from build123d import *

# Parameters (mm, degrees)
F0_W     = 19.05
F0_H     = 254
F1_DEPTH = 19.05
F0_W_2   = 241.3
F2_DEPTH = 12.7


with BuildPart() as f1:
    # F0 (on Front) → F1 (new body)
    with BuildSketch(Plane.XZ):
        with Locations((-269.875, 0)):
            Rectangle(F0_W, F0_H)
    extrude(amount=F1_DEPTH)



with BuildPart() as f1b:
    # F0 (on Front) → F1, piece 2 (new body)
    with BuildSketch(Plane.XZ):
        with Locations((-120.65, 0)):
            Rectangle(F0_W_2, F0_H)
        with Locations((120.65, 0)):
            Rectangle(F0_W_2, F0_H)
    extrude(amount=F1_DEPTH)


with BuildPart() as f1c:
    # F0 (on Front) → F1, piece 3 (new body)
    with BuildSketch(Plane.XZ):
        with Locations((269.875, 0)):
            Rectangle(F0_W, F0_H)
    extrude(amount=F1_DEPTH)


with BuildPart() as f1_1:
    add(f1.part)

    add(f1b.part)  # F2 merges F1b

    add(f1c.part)  # F2 merges F1c
    # F0 (on Front) → F2 (join)
    with BuildSketch(Plane.XZ):
        with Locations((-250.825, 0)):
            Rectangle(F0_W, F0_H)
        with Locations((250.825, 0)):
            Rectangle(F0_W, F0_H)
    extrude(amount=F2_DEPTH)


solid = f1_1.part
Verification items for the finished model (mm, model axes). A direction names the side the tool comes from. Coordinates: 2 decimals unless noted, no trailing zeros. Write each loop counter-clockwise with the first axis right and the second up, starting at its lowest first coordinate (ties: lowest second). Pieces come first, ordered by that corner, then holes. Notation, with made-up numbers: M -10,-31 L 39,-31 A21 ccw 39,-18 Z; hole C -33,-17 d10. An arc over 180 degrees is marked long. Use a Markdown table: item, result.
Q1. Thickness scan on line 1 (X direction, y = -14.25, z = 79); line 2 (Y direction, x = 243.5, z = -34.5). Record the ranges inside material, lowest first.
Reply:
| item | result |
|---|---|
| line 1 | x = -279.4 to -260.35, -241.3 to 241.3, 260.35 to 279.4 |
| line 2 | y = -12.7 to 0 |
Q2. Draft check along X on faces 3 (the face through (-279.4, -9, -2)), 4 (the face through (-251, -12.7, 2)), 5 (the face through (-3, -19.05, 2)). Enter one of: +X half, -X half, draft (parallel to the pull), parting line (faces both ways), or undercut.
Reply:
| item | result |
|---|---|
| face 3 | -X half |
| face 4 | undercut |
| face 5 | draft |
Q3. Sectioned sample at A-A, the plane y = -16. Record the boundary of the cut face in (x, z).
Reply:
| item | result |
|---|---|
| outline | M -279.4,-127 L -260.35,-127 L -260.35,127 L -279.4,127 Z; M -241.3,-127 L 241.3,-127 L 241.3,127 L -241.3,127 Z; M 260.35,-127 L 279.4,-127 L 279.4,127 L 260.35,127 Z |
Q4. Set-up check for faces 1 (the face through (251, -12.7, 2)), 2 (the face through (-4, -9, 127)): record each of +Z, -Z, +X, -X, +Y, -Y from which the full face is reachable in a straight line by a thin tool's end or side.
Reply:
| item | result |
|---|---|
| face 1 | +Z, -Z, -Y |
| face 2 | +Z, +X, -X, +Y, -Y |
Q5. Sectioned sample at B-B, the plane z = 66.5. Record the boundary of the cut face in (x, y).
Reply:
| item | result |
|---|---|
| outline | M -279.4,-19.05 L -260.35,-19.05 L -260.35,-12.7 L -241.3,-12.7 L -241.3,-19.05 L 241.3,-19.05 L 241.3,-12.7 L 260.35,-12.7 L 260.35,-19.05 L 279.4,-19.05 L 279.4,0 L -279.4,0 Z |
Q6. Go/stop test with a flat-tipped pin: P1, Ø15, axis at x = -249, z = -1.5, coming from the -Y side. Record where the tip stops, or that it passes through.
Reply:
| item | result |
|---|---|
| P1 | stops at y = -12.7 |
